```python
from build123d import *

# Parameters (mm, degrees)
SKETCH1_W                = 8.5
SKETCH1_H                = 56.8
BOSS_EXTRUDE1_DEPTH      = 4.75
M3_CLEARANCE_HOLE1_D     = 3.4
M3_CLEARANCE_HOLE1_DEPTH = 5
M3_CLEARANCE_HOLE1_TIP   = 1.021463052
SKETCH6_R                = 2.85
CUT_EXTRUDE1_DEPTH       = 2.2


with BuildPart() as part:
    # Sketch1 → Boss-Extrude1 (new body)
    with BuildSketch(Plane.XY):
        with Locations((4.25, -28.4)):
            Rectangle(SKETCH1_W, SKETCH1_H)
    extrude(amount=BOSS_EXTRUDE1_DEPTH)

    # M3 Clearance Hole1
    with Locations(Plane.XY.offset(4.75)):
        with Locations((4.25, -16.7), (4.25, -40.1)):
            Hole(M3_CLEARANCE_HOLE1_D / 2, depth=M3_CLEARANCE_HOLE1_DEPTH)
            with Locations((0, 0, -(M3_CLEARANCE_HOLE1_DEPTH + M3_CLEARANCE_HOLE1_TIP / 2))):  # 118° drill point
                Cone(0, M3_CLEARANCE_HOLE1_D / 2, M3_CLEARANCE_HOLE1_TIP, mode=Mode.SUBTRACT)

    # Sketch6 → Cut-Extrude1 (cut)
    with BuildSketch(Plane.XY.offset(4.75)):
        with Locations((4.25, -16.7)):
            Circle(SKETCH6_R)
        with Locations((4.25, -40.1)):
            Circle(SKETCH6_R)
    extrude(amount=-CUT_EXTRUDE1_DEPTH, mode=Mode.SUBTRACT)


solid = part.part
```
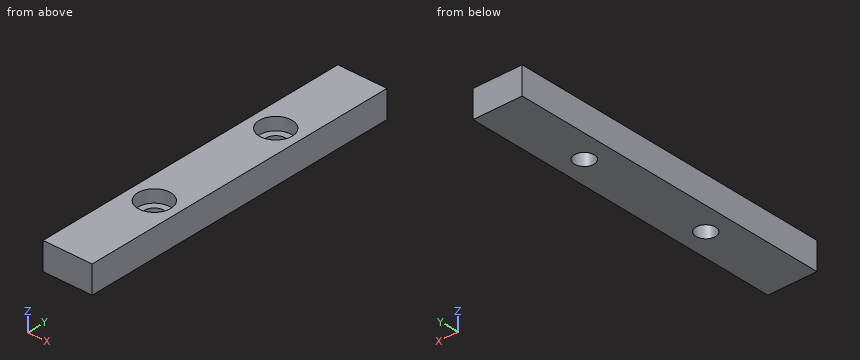
Input: part model. Units: mm. Frame: model coordinates. Round coordinates to 2 decimals unless told otherwise and drop trailing zeros. Write each loop counter-clockwise with the first axis right and the second up, starting at its lowest first coordinate (ties: lowest second). Pieces come first, ordered by that corner, then holes. Notation, with made-up numbers: M -21.75,47.5 L 0.25,47.5 A21 cw 0.25,55.5 Z; hole C 43,-29 d10. An arc over 180 degrees is marked long. Write each question's results on one line, items separated by ' | '.
Q1. Section query A-A (x = 4.25). Return loops of the section in (y, z), and give its area (3 significant figures).
Results:
outline: M -56.8,0 L -41.8,0 L -41.8,2.55 L -42.95,2.55 L -42.95,4.75 L -56.8,4.75 Z; M -38.4,0 L -18.4,0 L -18.4,2.55 L -19.55,2.55 L -19.55,4.75 L -37.25,4.75 L -37.25,2.55 L -38.4,2.55 Z; M -15,0 L 0,0 L 0,4.75 L -13.85,4.75 L -13.85,2.55 L -15,2.55 Z | area: 227 mm^2
Q2. Pin query (flat end, axial travel): P1, Ø4.5, axis at x = 4.25, y = -40.1, coming from the +Z side; P2, Ø2, axis at x = 4.25, y = -16.7, coming from the -Z side; P3, Ø4, axis at x = 5.5, y = -11, coming from the -Z side. Return the tip coordinate at first contact, or that it passes through.
Results:
P1: stops at z = 2.55 | P2: passes through | P3: stops at z = 0
Q3. Line query: line 1 along Y through (x, z) = (4.25, 3.1); line 2 along Y through (x, z) = (4.25, 0.6); line 3 along X through (y, z) = (-17, 2.6). Output: solid intervals per line, ascending.
Results:
line 1: y = -56.8 to -42.95, -37.25 to -19.55, -13.85 to 0 | line 2: y = -56.8 to -41.8, -38.4 to -18.4, -15 to 0 | line 3: x = 0 to 1.42, 7.08 to 8.5
Q4. Section query D-D (z = 3.7). Return loops of the section in (x, y).
Results:
outline: M 0,-56.8 L 8.5,-56.8 L 8.5,0 L 0,0 Z; hole C 4.25,-40.1 d5.7; hole C 4.25,-16.7 d5.7
Q5. Section query B-B (y = -40.1). Return loops of the section in (x, z).
Results:
outline: M 0,0 L 2.55,0 L 2.55,2.55 L 1.4,2.55 L 1.4,4.75 L 0,4.75 Z; M 5.95,0 L 8.5,0 L 8.5,4.75 L 7.1,4.75 L 7.1,2.55 L 5.95,2.55 Z
Q6. Section query C-C (z = 1.25). Return loops of the section in (x, y), and give its area (3 significant figures).
Results:
outline: M 0,-56.8 L 8.5,-56.8 L 8.5,0 L 0,0 Z; hole C 4.25,-40.1 d3.4; hole C 4.25,-16.7 d3.4 | area: 465 mm^2
